from build123d import *

# Parameters (mm, degrees)
SKETCH4_W           = 51.6
SKETCH4_H           = 23.6
SKETCH4_W_2         = 50
SKETCH4_H_2         = 22
BOSS_EXTRUDE2_DEPTH = 24.2
SKETCH4_2_W         = 50
SKETCH4_2_H         = 22
BOSS_EXTRUDE3_DEPTH = 0.8
FILLET3_R           = 3.18
FILLET4_R           = 0.5


with BuildPart() as part:
    # Sketch4 → Boss-Extrude2 (new body)
    with BuildSketch(Plane(origin=(0, 0, 0), x_dir=(1, 0, 0), z_dir=(0, 1, 0))):
        Rectangle(SKETCH4_W, SKETCH4_H)
        Rectangle(SKETCH4_W_2, SKETCH4_H_2, mode=Mode.SUBTRACT)
    extrude(amount=BOSS_EXTRUDE2_DEPTH)

    # Sketch4<2> → Boss-Extrude3 (add)
    with BuildSketch(Plane(origin=(0, 0, 0), x_dir=(1, 0, 0), z_dir=(0, 1, 0))):
        Rectangle(SKETCH4_2_W, SKETCH4_2_H)
    extrude(amount=BOSS_EXTRUDE3_DEPTH)

    # Fillet3
    fillet3_edges = [part.edges().sort_by_distance(p)[0] for p in [
        (-25, 12.5, -11),
        (-25, 12.5, 11),
        (25, 12.5, 11),
        (25, 12.5, -11),
        (25.8, 12.1, 11.8),
        (-25.8, 12.1, 11.8),
        (-25.8, 12.1, -11.8),
        (25.8, 12.1, -11.8),
    ]]
    fillet(fillet3_edges, radius=FILLET3_R)

    # Fillet4
    fillet4_edges = [part.edges().sort_by_distance(p)[0] for p in [
        (25.8, 0, 0),
        (0, 0, 11.8),
        (-25.8, 0, 0),
        (0, 0, -11.8),
        (-24.868599564, 0, -10.868599564),
        (-24.868599564, 0, 10.868599564),
        (24.868599564, 0, -10.868599564),
        (24.868599564, 0, 10.868599564),
        (25, 0.8, 0),
        (0, 0.8, -11),
        (-25, 0.8, 0),
        (0, 0.8, 11),
        (24.068599564, 0.8, 10.068599564),
        (-24.068599564, 0.8, -10.068599564),
        (-24.068599564, 0.8, 10.068599564),
        (24.068599564, 0.8, -10.068599564),
    ]]
    fillet(fillet4_edges, radius=FILLET4_R)


solid = part.part
Part model, mm, in its own coordinate system. A direction names the side the tool comes from. Round coordinates to 2 decimals unless told otherwise and drop trailing zeros. Write each loop counter-clockwise with the first axis right and the second up, starting at its lowest first coordinate (ties: lowest second). Pieces come first, ordered by that corner, then holes. Notation, with made-up numbers: (9, 77.25) - (24, 77.25) arc R3 cw to (24, 82.25) - close; hole circle Ø7 at (-23, 63). An arc over 180 degrees is marked (long way). Use CSV: the item, a comma, the result in double quotes.
Item 1: Flat gauge pin, fed straight in: P1, Ø5, axis at x = -7, z = -4.5, coming from the +Y side. Where does the tip first touch, or does it go through?
Results list:
P1,"stops at y = 0.8"
Item 2: Slice it at A-A, the plane z = 6. Write the cut outline in (x, y).
Results list:
outline,"(-25.8, 0.5) arc R0.5 ccw to (-25.3, 0) - (25.3, 0) arc R0.5 ccw to (25.8, 0.5) - (25.8, 24.2) - (25, 24.2) - (25, 1.3) arc R0.5 cw to (24.5, 0.8) - (-24.5, 0.8) arc R0.5 cw to (-25, 1.3) - (-25, 24.2) - (-25.8, 24.2) - close"
Item 3: Tool access for faces 1 (the cylindrical face through (-24.893, 12.516, 10.844)), 2 (the cylindrical face through (-24.044, 12.91, -10.093)): list every direction of +Z, -Z, +X, -X, +Y, -Y with a clear straight run to the whole face (end or side of a thin tool).
Results list:
face 1,"+Z, -X, +Y, -Y"
face 2,"+Y"
Item 4: Slice it at B-B, the plane y = 3.75. Write the cut outline in (x, z).
Results list:
outline,"(-25.8, -8.62) arc R3.18 ccw to (-22.62, -11.8) - (22.62, -11.8) arc R3.18 ccw to (25.8, -8.62) - (25.8, 8.62) arc R3.18 ccw to (22.62, 11.8) - (-22.62, 11.8) arc R3.18 ccw to (-25.8, 8.62) - close; hole (-25, -7.82) arc R3.18 ccw to (-21.82, -11) - (21.82, -11) arc R3.18 ccw to (25, -7.82) - (25, 7.82) arc R3.18 ccw to (21.82, 11) - (-21.82, 11) arc R3.18 ccw to (-25, 7.82) - close"
Item 5: Wall check: L1, parallel to Z at x = 12.5, y = 2.5; L2, parallel to X at y = 10.5, z = -0.75; L3, parallel to Y at x = -12, z = -7.5. Give the ranges that are in metal, low to high.
Results list:
L1,"z = -11.8 to -11, 11 to 11.8"
L2,"x = -25.8 to -25, 25 to 25.8"
L3,"y = 0 to 0.8"
Item 6: Pull direction Z, two halves, no side cores. Call faces 3 (the cylindrical face through (24.844, 12.516, -10.893)), 4 (the flat face through (-0.1, 24.2, -11.4)), 5 (the flat face through (25, 13, 0)): pulls with the +Z half, pulls with the -Z half, needs draft (parallel to the pull), parting line crosses it, or undercut.
Results list:
face 3,"pulls with the -Z half"
face 4,"needs draft"
face 5,"undercut"
Item 7: Slice it at C-C, the plane x = 19.5. Write the cut outline in (y, z).
Results list:
outline,"(0, -11.3) arc R0.5 ccw to (0.5, -11.8) - (24.2, -11.8) - (24.2, -11) - (1.3, -11) arc R0.5 cw to (0.8, -10.5) - (0.8, 10.5) arc R0.5 cw to (1.3, 11) - (24.2, 11) - (24.2, 11.8) - (0.5, 11.8) arc R0.5 ccw to (0, 11.3) - close"
